```python
from build123d import *

# Parameters (mm, degrees)
SKETCH1_R             = 4.75
SKETCH1_R_2           = 2.2
BOSS_EXTRUDE1_DEPTH   = 2
SKETCH1_R_3           = 1.275
BOSS_EXTRUDE1_2_DEPTH = 2
SKETCH1_3_R           = 2.2
SKETCH1_3_R_2         = 1.275
BOSS_EXTRUDE2_DEPTH   = 4.25


with BuildPart() as part:
    # Sketch1 → Boss-Extrude1 (new body)
    with BuildSketch(Plane.XY):
        Circle(SKETCH1_R)
        Circle(SKETCH1_R_2, mode=Mode.SUBTRACT)
    extrude(amount=BOSS_EXTRUDE1_DEPTH)



with BuildPart() as body_2:
    # Sketch1 → Boss-Extrude1 2 (new body)
    with BuildSketch(Plane.XY):
        Circle(SKETCH1_R_3)
    extrude(amount=BOSS_EXTRUDE1_2_DEPTH)


with BuildPart() as part_1:
    add(part.part)

    add(body_2.part)  # Boss-Extrude2 merges body 2
    # Sketch1<3> → Boss-Extrude2 (add)
    with BuildSketch(Plane.XY):
        Circle(SKETCH1_3_R)
        Circle(SKETCH1_3_R_2, mode=Mode.SUBTRACT)
    extrude(amount=BOSS_EXTRUDE2_DEPTH)


solid = part_1.part
```
Input: part model. Units: mm. Frame: model coordinates. A direction names the side the tool comes from. Round coordinates to 2 decimals unless told otherwise and drop trailing zeros. Loops run counter-clockwise (first coordinate to the right, second up) from the corner with the lowest first, then second, coordinate; pieces in that order, holes last.
1) Section query D-D on z = 1.1. Return the cut outline in (x, y).
Ans:
outline: circle Ø9.5 at (0, 0)
2) Section query A-A on x = 0. Return the cut outline in (y, z) (3 decimals), plus the area to 3 significant figures.
Ans:
outline: (-4.75, 0) - (4.75, 0) - (4.75, 2) - (2.2, 2) - (2.2, 4.25) - (1.275, 4.25) - (1.275, 2) - (-1.275, 2) - (-1.275, 4.25) - (-2.2, 4.25) - (-2.2, 2) - (-4.75, 2) - close
area: 23.2 mm2
3) Pull-direction query (Y, two-part tool) for faces 3 (the flat face through (0, 0, 2)), 4 (the flat face through (-0.03, -1.44, 4.25)), 5 (the cylindrical face through (2.1, 0.66, 3.11)); classes: released by +Y, released by -Y, zero draft, split by the parting line, or undercut.
Ans:
face 3: undercut
face 4: zero draft
face 5: split by the parting line
4) Pin query (flat end, axial travel): pin 1 (1 mm diameter, centred on y = -0.5, z = 1.5, fed in from -X); pin 2 (2 mm diameter, centred on x = 2, z = 2, fed in from +Y). Return the tip coordinate at first contact, or that it passes through.
Ans:
pin 1: stops at x = -4.75
pin 2: stops at y = 4.64
5) Section query C-C on z = 2.45. Return the cut outline in (x, y) (3 decimals).
Ans:
outline: circle Ø4.4 at (0, 0); hole circle Ø2.55 at (0, 0)
6) Set-up query: faces 1 (the cylindrical face through (0.59, -1.13, 3.11)), 2 (the cylindrical face through (2.192, -4.214, 0.986)). Return all of +Z, -Z, +X, -X, +Y, -Y with unobstructed straight access to the full face (end or side cutting, diameter ignored); none if empty.
Ans:
face 1: +Z
face 2: +Z, -Z
7) Material intervals for line 1 (Y direction, x = 0, z = 2.6) (3 decimals); line 2 (Z direction, x = 0, y = 3.25); line 3 (X direction, y = -0.75, z = 0.4), sorted ascending.
Ans:
line 1: y = -2.2 to -1.275, 1.275 to 2.2
line 2: z = 0 to 2
line 3: x = -4.69 to 4.69
